For this review, take the finished solid that the model builds, in its own axes (mm). A direction names the side the tool comes from. Give positions to 0.01 mm unless a question says otherwise; leave off trailing zeros. Order: outer loops, then holes, each group sorted by start corner. A loop starts at its lowest first (then second) coordinate and runs counter-clockwise, first axis right, second up. Notation, with made-up numbers: (53.5, 44) - (71.5, 44) arc R24 ccw to (71.5, 57) - close; hole circle Ø5 at (51.25, 66.25). An arc over 180 degrees is marked (long way). Answer as a JSON object with one key per item and string values. Group by question number.
from build123d import *

# Parameters (mm, degrees)
ESQUISSE1_W             = 16.5
ESQUISSE1_H             = 1.6
ESQUISSE2_R             = 37.6
ESQUISSE2_R_2           = 35
ENL_V_MAT_EXTRU_1_DEPTH = 0.1


with BuildPart() as part:
    # Esquisse1 → Révolution1 (revolve)
    with BuildSketch(Plane.XY, mode=Mode.PRIVATE) as r_volution1_sk:
        with Locations((30.75, 0)):
            Rectangle(ESQUISSE1_W, ESQUISSE1_H)
    revolve(r_volution1_sk.sketch.rotate(Axis((0, -15.298646519, 0), (0, 1, 0)), 90), axis=Axis((0, -15.298646519, 0), (0, 1, 0)))

    # Esquisse2 → Enlèv. mat.-Extru.1 (cut)
    with BuildSketch(Plane(origin=(0, 0.8, 0), x_dir=(1, 0, 0), z_dir=(0, 1, 0))):
        with Locations(Location((0, 0, 0), (0, 0, 270))):
            Circle(ESQUISSE2_R)
        with Locations(Location((0, 0, 0), (0, 0, 270))):
            Circle(ESQUISSE2_R_2, mode=Mode.SUBTRACT)
    extrude(amount=-ENL_V_MAT_EXTRU_1_DEPTH, mode=Mode.SUBTRACT)


solid = part.part
1) Consider section A-A (x = 0). Give the boundary of the cut face in (y, z).
2) For line 1 (X direction, y = -0.3, z = 0); line 2 (Z direction, x = -6, y = -0.55); line 3 (Z direction, x = 15.5, y = 0.35), list the stretches that pass through material, from the lowest coordinate up.
3) Consider section C-C (z = 31). Give the boundary of the cut face in (x, y).
4) Mouldability with a two-part tool opening along X and no side actions: class faces 3 (the face through (-38.668, 0.011, 5.077)), 4 (the face through (17, -0.8, 17)), 5 (the face through (19.961, 0.011, -10.382)) as released by +X, released by -X, zero draft, split by the parting line, or undercut.
5) For faces 1 (the face through (23, 0.8, 0)), 2 (the face through (-25, 0.7, 25)), list the 3-axis set-ups (+Z, -Z, +X, -X, +Y, -Y) from which the entire face can be reached by the end or side of a thin tool; tool diameter is ignored.
6) Consider section B-B (z = 0). Give the boundary of the cut face in (x, y), plus the area to 3 significant figures.
7) Consider section D-D (y = -0.45). Give the boundary of the cut face in (x, z).
Result set:
{
 "1": {"outline": "(-0.8, -39) - (0.8, -39) - (0.8, -37.6) - (0.7, -37.6) - (0.7, -35) - (0.8, -35) - (0.8, -22.5) - (-0.8, -22.5) - close; (-0.8, 22.5) - (0.8, 22.5) - (0.8, 35) - (0.7, 35) - (0.7, 37.6) - (0.8, 37.6) - (0.8, 39) - (-0.8, 39) - close"},
 "2": {"line 1": "x = -39 to -22.5, 22.5 to 39", "line 2": "z = -38.54 to -21.69, 21.69 to 38.54", "line 3": "z = -35.79 to -16.31, 16.31 to 35.79"},
 "3": {"outline": "(-23.66, -0.8) - (23.66, -0.8) - (23.66, 0.8) - (21.28, 0.8) - (21.28, 0.7) - (16.25, 0.7) - (16.25, 0.8) - (-16.25, 0.8) - (-16.25, 0.7) - (-21.28, 0.7) - (-21.28, 0.8) - (-23.66, 0.8) - close"},
 "4": {"face 3": "split by the parting line", "face 4": "zero draft", "face 5": "undercut"},
 "5": {"face 1": "+Z, -Z, +X, -X, +Y", "face 2": "+Y"},
 "6": {"outline": "(-39, -0.8) - (-22.5, -0.8) - (-22.5, 0.8) - (-35, 0.8) - (-35, 0.7) - (-37.6, 0.7) - (-37.6, 0.8) - (-39, 0.8) - close; (22.5, -0.8) - (39, -0.8) - (39, 0.8) - (37.6, 0.8) - (37.6, 0.7) - (35, 0.7) - (35, 0.8) - (22.5, 0.8) - close", "area": "52.3 mm2"},
 "7": {"outline": "circle Ø78 at (0, 0); hole circle Ø45 at (0, 0)"}
}
